from build123d import *

# Parameters (mm, degrees)
SKETCH1_R           = 88.9
BOSS_EXTRUDE1_DEPTH = 12.7
SKETCH9_W           = 49.53
SKETCH9_H           = 49.53
SKETCH9_W_2         = 44.45
SKETCH9_H_2         = 44.45
BOSS_EXTRUDE2_DEPTH = 19.05
SKETCH10_R          = 5.715
CUT_EXTRUDE7_DEPTH  = 0.508
SKETCH14_R          = 19.05
CUT_EXTRUDE11_DEPTH = 12.7
SKETCH15_R          = 12.7
SKETCH15_R_2        = 6.35
BOSS_EXTRUDE3_DEPTH = 25.4
CUT_EXTRUDE12_START = -12.7
SKETCH16_R          = 6.35
CUT_EXTRUDE12_DEPTH = 12.7
SKETCH17_R          = 9.525
CUT_EXTRUDE13_DEPTH = 25.4
CHAMFER2_SIZE       = 2.54
CHAMFER2_SIZE2      = 4.399409051
SKETCH19_R          = 12.7
SKETCH19_R_2        = 1.524
CUT_EXTRUDE14_DEPTH = 12.7
CUT_EXTRUDE15_START = -5.08
SKETCH21_R          = 4.064
SKETCH21_R_2        = 5.715
CUT_EXTRUDE15_DEPTH = 5.08
SKETCH22_W          = 52.07
SKETCH22_H          = 26.162
CUT_EXTRUDE17_DEPTH = 3.81
BOSS_EXTRUDE5_START = -7.62
BOSS_EXTRUDE5_DEPTH = 7.62
FILLET2_R           = 5.08


with BuildPart() as part:
    # Sketch1 → Boss-Extrude1 (new body)
    with BuildSketch(Plane(origin=(0, 0, 0), x_dir=(1, 0, 0), z_dir=(0, 1, 0))):
        with Locations(Location((0, 0, 0), (0, 0, 270))):
            Circle(SKETCH1_R)
    extrude(amount=BOSS_EXTRUDE1_DEPTH)

    # Sketch9 → Boss-Extrude2 (add)
    with BuildSketch(Plane(origin=(0, 12.7, 0), x_dir=(1, 0, 0), z_dir=(0, 1, 0))):
        with Locations((0, 56.134)):
            Rectangle(SKETCH9_W, SKETCH9_H)
        with Locations((0, 56.134)):
            Rectangle(SKETCH9_W_2, SKETCH9_H_2, mode=Mode.SUBTRACT)
    extrude(amount=BOSS_EXTRUDE2_DEPTH)

    # Sketch10 → Cut-Extrude7 (cut)
    with BuildSketch(Plane(origin=(0, 12.7, 0), x_dir=(1, 0, 0), z_dir=(0, 1, 0))):
        with Locations(Location((-71.490397082, -41.275, 0), (0, 0, 270))):
            Circle(SKETCH10_R)
        with Locations(Location((-71.490397082, 41.275, 0), (0, 0, 270))):
            Circle(SKETCH10_R)
        with Locations(Location((71.490397082, 41.275, 0), (0, 0, 270))):
            Circle(SKETCH10_R)
        with Locations(Location((71.490397082, -41.275, 0), (0, 0, 270))):
            Circle(SKETCH10_R)
    extrude(amount=-CUT_EXTRUDE7_DEPTH, mode=Mode.SUBTRACT)

    # Sketch14 → Cut-Extrude11 (cut)
    with BuildSketch(Plane.XZ):
        with Locations(Location((0, 0, 0), (0, 0, 270))):
            Circle(SKETCH14_R)
    extrude(amount=-CUT_EXTRUDE11_DEPTH, mode=Mode.SUBTRACT)

    # Sketch15 → Boss-Extrude3 (add)
    # profile 1 of 2: a face of its own
    with BuildSketch(Plane(origin=(0, 12.7, 0), x_dir=(1, 0, 0), z_dir=(0, 1, 0))):
        with Locations(Location((-41.275, 0, 0), (0, 0, 270))):
            Circle(SKETCH15_R)
        with Locations(Location((-41.275, 0, 0), (0, 0, 270))):
            Circle(SKETCH15_R_2, mode=Mode.SUBTRACT)
    # profile 2 of 2: a face of its own
    with BuildSketch(Plane(origin=(0, 12.7, 0), x_dir=(1, 0, 0), z_dir=(0, 1, 0))):
        with Locations(Location((41.275, 0, 0), (0, 0, 270))):
            Circle(SKETCH15_R)
        with Locations(Location((41.275, 0, 0), (0, 0, 270))):
            Circle(SKETCH15_R_2, mode=Mode.SUBTRACT)
    extrude(amount=BOSS_EXTRUDE3_DEPTH)

    # Sketch16 → Cut-Extrude12 (cut)
    with BuildSketch(Plane(origin=(0, 12.7, 0), x_dir=(1, 0, 0), z_dir=(0, 1, 0)).offset(CUT_EXTRUDE12_START)):
        with Locations(Location((41.275, 0, 0), (0, 0, 270))):
            Circle(SKETCH16_R)
        with Locations(Location((-41.275, 0, 0), (0, 0, 270))):
            Circle(SKETCH16_R)
    extrude(amount=CUT_EXTRUDE12_DEPTH, mode=Mode.SUBTRACT)

    # Sketch17 → Cut-Extrude13 (cut)
    with BuildSketch(Plane.XZ):
        with Locations(Location((41.275, 0, 0), (0, 0, 270))):
            Circle(SKETCH17_R)
        with Locations(Location((-41.275, 0, 0), (0, 0, 270))):
            Circle(SKETCH17_R)
    extrude(amount=-CUT_EXTRUDE13_DEPTH, mode=Mode.SUBTRACT)

    # Chamfer2
    chamfer2_edges = [part.edges().sort_by_distance(p)[0] for p in [
        (-41.275, 12.7, -12.7),
        (41.275, 12.7, -12.7),
    ]]
    chamfer2_side = [part.faces().sort_by_distance(p)[0] for p in [
        (0, 12.7, -86.385528286),
    ]]
    chamfer(chamfer2_edges, length=CHAMFER2_SIZE, length2=CHAMFER2_SIZE2, reference=chamfer2_side[0])

    # Sketch19 → Cut-Extrude14 (cut)
    with BuildSketch(Plane(origin=(0, 12.7, 0), x_dir=(1, 0, 0), z_dir=(0, 1, 0))):
        with Locations(Location((0, 56.134, 0), (0, 0, 270))):
            Circle(SKETCH19_R)
        with Locations(Location((15.494, 71.628, 0), (0, 0, 270))):
            Circle(SKETCH19_R_2)
        with Locations(Location((15.494, 40.64, 0), (0, 0, 270))):
            Circle(SKETCH19_R_2)
        with Locations(Location((-15.494, 40.64, 0), (0, 0, 270))):
            Circle(SKETCH19_R_2)
        with Locations(Location((-15.494, 71.628, 0), (0, 0, 270))):
            Circle(SKETCH19_R_2)
    extrude(amount=-CUT_EXTRUDE14_DEPTH, mode=Mode.SUBTRACT)

    # Sketch21 → Cut-Extrude15 (cut)
    with BuildSketch(Plane.XZ.offset(CUT_EXTRUDE15_START)):
        with Locations(Location((-15.494, -71.628, 0), (0, 0, 270))):
            Circle(SKETCH21_R)
        with Locations(Location((15.494, -71.628, 0), (0, 0, 270))):
            Circle(SKETCH21_R)
        with Locations(Location((15.494, -40.64, 0), (0, 0, 270))):
            Circle(SKETCH21_R)
        with Locations(Location((-15.494, -40.64, 0), (0, 0, 270))):
            Circle(SKETCH21_R)
        with Locations(Location((-71.490397082, 41.275, 0), (0, 0, 90))):
            Circle(SKETCH21_R_2)
        with Locations(Location((71.490397082, 41.275, 0), (0, 0, 90))):
            Circle(SKETCH21_R_2)
        with Locations(Location((71.490397082, -41.275, 0), (0, 0, 90))):
            Circle(SKETCH21_R_2)
        with Locations(Location((-71.490397082, -41.275, 0), (0, 0, 90))):
            Circle(SKETCH21_R_2)
    extrude(amount=CUT_EXTRUDE15_DEPTH, mode=Mode.SUBTRACT)

    # Sketch22 → Cut-Extrude17 (cut)
    with BuildSketch(Plane(origin=(0, 12.7, 0), x_dir=(1, 0, 0), z_dir=(0, 1, 0))):
        with Locations((0, -48.641)):
            Rectangle(SKETCH22_W, SKETCH22_H)
    extrude(amount=-CUT_EXTRUDE17_DEPTH, mode=Mode.SUBTRACT)

    # Sketch23 → Boss-Extrude5 (add)
    with BuildSketch(Plane(origin=(0, 12.7, 0), x_dir=(1, 0, 0), z_dir=(0, 1, 0)).offset(BOSS_EXTRUDE5_START)):
        with BuildLine():
            Line((-38.1, -80.321852568), (-38.1, -127))
            Line((-38.1, -127), (38.1, -127))
            Line((38.1, -127), (38.1, -80.321852568))
            ThreePointArc((38.1, -80.321852568), (0, -88.9), (-38.1, -80.321852568))
        make_face()
    extrude(amount=BOSS_EXTRUDE5_DEPTH)

    # Fillet2
    fillet2_edges = [part.edges().sort_by_distance(p)[0] for p in [
        (-19.526870034, 5.08, 86.728953335),
        (-38.1, 8.89, 80.321852568),
        (38.1, 8.89, 80.321852568),
        (38.1, 8.89, 127),
        (-38.1, 8.89, 127),
    ]]
    fillet(fillet2_edges, radius=FILLET2_R - 0.0001)  # a hair under: the kernel refuses the full size


solid = part.part
Geometry check sheet. Reference: the model listing, model coordinates, mm. A direction names the side the tool comes from. Give positions to 0.01 mm unless a question says otherwise; leave off trailing zeros. Order: outer loops, then holes, each group sorted by start corner. A loop starts at its lowest first (then second) coordinate and runs counter-clockwise, first axis right, second up. Notation, with made-up numbers: (54, 44) - (90, 44) arc R22 cw to (90, 66) - close; hole circle Ø8 at (-10, -6.75). An arc over 180 degrees is marked (long way). Use one line per item in the form item = value.
1) Depth check by flat-ended pin: pin 1 Ø5 at (y, z) = (10, 63.5) entering from -X; pin 2 Ø5.5 at (x, z) = (70, 40) entering from +Y; pin 3 Ø5 at (x, y) = (-8, 19) entering from +Z. Enter the tip coordinate at first touch or a pass-through.
Working result:
pin_1 = -64.67
pin_2 = 12.19
pin_3 = -31.37
2) Sectioned sample at B-B (z = -60). Record the boundary of the cut face in (x, y) (3 decimals), and give its area (3 significant figures).
Working result:
outline = (-65.599, 0) - (-12.097, 0) - (-12.097, 12.7) - (-22.225, 12.7) - (-22.225, 31.75) - (-24.765, 31.75) - (-24.765, 12.7) - (-65.599, 12.7) - close; (12.097, 0) - (65.599, 0) - (65.599, 12.7) - (24.765, 12.7) - (24.765, 31.75) - (22.225, 31.75) - (22.225, 12.7) - (12.097, 12.7) - close
area = 1,460 mm^2
3) Material ranges on probe 1 along X at (y, z) = (8, 0); probe 2 along Z at (x, y) = (-6.5, 15.5); probe 3 along X at (y, z) = (29.5, 3.5), recorded low to high. Write a range as from..to.
Working result:
probe_1 = -88.9..-50.8, -31.75..-19.05, 19.05..31.75, 50.8..88.9
probe_2 = -80.9..-78.36, -33.91..-31.37
probe_3 = -53.48..-46.57, -35.98..-29.07, 29.07..35.98, 46.57..53.48
4) Sectioned sample at D-D (x = -60). Record the boundary of the cut face in (y, z).
Working result:
outline = (0, -65.6) - (12.7, -65.6) - (12.7, 65.6) - (0, 65.6) - close
5) Sectioned sample at A-A (x = 0). Count the separate pieces of the cut face and the enclosed holes in it, and give its area (3 significant figures).
Working result:
separate_pieces = 3
enclosed_holes = 0
area = 1,740 mm^2
6) Draft check along Z on faces 6 (the face through (-31.83, 12.52, 1.24)), 7 (the face through (19, 12.7, 18)), 8 (the face through (0, 9, 127)). Enter one of: released by +Z, released by -Z, zero draft, split by the parting line, or undercut.
Working result:
face_6 = undercut
face_7 = zero draft
face_8 = released by +Z
7) Access from +Z, -Z, +X, -X, +Y, -Y to the whole of each face (thin tool, end or side, straight path). Record for faces 1 (the face through (0, 22, -31.369)), 2 (the face through (-38.1, 9, 102)), 3 (the face through (-17.967, 2.576, -37.415)), 4 (the face through (-47.474, 31.661, -1.377)), 5 (the face through (28.877, 27.453, -2.753)).
Working result:
face_1 = +Z, +X, -X, +Y
face_2 = +Z, -X, +Y, -Y
face_3 = -Y
face_4 = +Y, -Y
face_5 = +Y
